Autodesk Inventor part; units mm, degrees
ref_plane "YZ Plane" through (0, 0, 0) normal (1, 0, 0) x (0, 1, 0)
ref_plane "XZ Plane" through (0, 0, 0) normal (0, 1, 0) x (-1, 0, 0)
ref_plane "XY Plane" through (0, 0, 0) normal (0, 0, 1) x (1, 0, 0)
sketch "Sketch1" plane through (0, 0, 0) normal (0, 0, 1) x (1, 0, 0)
  circle A0 centre (0, 0) radius 95.25
  dimension "d0" = 190.5
extrude "Extrusion1" add sketch "Sketch1" along normal blind 457.2
fillet "Fillet1" radius 25.4 1 edges at (-95.25, 0, 0)
fillet "Fillet2" radius 25.4 1 edges at (-95.25, 0, 457.2)
properties part number "daGasContiner"
Here's how the part is built. I have some questions about the finished solid (model axes, mm). Round coordinates to 2 decimals unless told otherwise and drop trailing zeros. Write each loop counter-clockwise with the first axis right and the second up, starting at its lowest first coordinate (ties: lowest second). Pieces come first, ordered by that corner, then holes.
Q1. Will these pins go through, and if not, where does the flat tip stop? P1, Ø6, axis at x = -54.5, y = 60.5, coming from the -Z side; P2, Ø5, axis at x = -63, z = 384.5, coming from the -Y side; P3, Ø6, axis at x = -69.5, y = -71.5, coming from the -Z side; P4, Ø2, axis at x = -18.5, z = 52, coming from the +Y side.
Q2. If we section it at A-A on z = 305.5: Write out the boundary of the cut face in (x, y).
Q3. Please list where these lines run through material, in increasing order: probe 1 along X at (y, z) = (1, 176.5); probe 2 along Z at (x, y) = (66, -27); probe 3 along X at (y, z) = (79.5, 407.5).
Answer below:
1. P1: stops at z = 1.49
1. P2: stops at y = -73.57
1. P3: passes through
1. P4: stops at y = 93.63
2. outline: circle Ø190.5 at (0, 0)
3. probe 1: x = -95.24 to 95.24
3. probe 2: z = 0.04 to 457.16
3. probe 3: x = -52.46 to 52.46
